Here's how the part is built. I have some questions about the finished solid (model axes, mm). A direction names the side the tool comes from. Coordinates: 2 decimals unless noted, no trailing zeros. Loops run counter-clockwise (first coordinate to the right, second up) from the corner with the lowest first, then second, coordinate; pieces in that order, holes last. Notation, with made-up numbers: M -31,45.5 L 19,45.5 A18 ccw 19,74.5 Z; hole C 37,-16 d2. An arc over 180 degrees is marked long. Use one line per item in the form item = value. Start each with the question number.
(1) Please list where these lines run through material, in increasing order: L1, parallel to X at y = 0.3, z = -0.55; L2, parallel to X at y = -1, z = 1.25; L3, parallel to Y at x = -4.7, z = -0.65.
(2) Imagine slicing it at C-C, the plane y = 0.3. Please give me the cut outline in (x, z), and give its area (3 significant figures).
(3) Thinking about a two-plate mould opening in Y: for faces 1 (the flat face through (0.4, 2.4, 4)), 2 (the flat face through (6.855, -2.158, -1.479)), 3 (the flat face through (0, 2, 7)), which applies, +Y half, -Y half, draft (parallel to the pull), parting line (faces both ways), or undercut?
(4) On a 3-axis mill with a long thin cutter (end or side, diameter ignored), from which of +Z, -Z, +X, -X, +Y, -Y can I reach the whole of each face in a straight line? I mean faces 4 (the flat face through (-6, 1, 0)), 5 (the flat face through (-4, -1.6, -1)), 6 (the flat face through (-1, 2, 1)). Say none if no direction works.
(5) Will these pins go through, and if not, where does the flat tip stop? P1, Ø2.5, axis at x = -4.5, z = -1, coming from the -Y side; P2, Ø1.7, axis at x = 4, y = 0, coming from the +Z side; P3, Ø4, axis at x = 3, z = 4.5, coming from the -Y side.
(6) Imagine slicing it at D-D, the plane z = 3.25. Please give me the cut outline in (x, y).
(7) Imagine slicing it at A-A, the plane x = -4.7. Please give me the cut outline in (y, z), and give its area (3 significant figures).
(8) Imagine slicing it at B-B, the plane z = -1.5. Please give me the cut outline in (x, y).
```python
from build123d import *

# Parameters (mm, degrees)
F1_DEPTH  = 7
F2_W      = 15.6
F2_H      = 6.4
F3_DEPTH  = 3
F5_DEPTH  = 1
F6_SIZE2  = 0.2
F6_SIZE   = 0.6
F8_DEPTH  = 3
F9_R      = 1.1
F10_DEPTH = 3


with BuildPart() as f1:
    # F0 (on Top) → F1 (new body)
    with BuildSketch(Plane.XY):
        with BuildLine():
            Line((-0.4, 2.9), (-0.4, 1.9595917942))
            ThreePointArc((-0.4, 1.9595917942), (0, -2), (0.4, 1.9595917942))
            Line((0.4, 1.9595917942), (0.4, 2.9))
            Line((0.4, 2.9), (5.4, 2.9))
            ThreePointArc((5.4, 2.9), (6.8142135624, 2.3142135624), (7.4, 0.9))
            Line((7.4, 0.9), (7.4, -2.7))
            Line((7.4, -2.7), (7.8, -2.7))
            Line((7.8, -2.7), (7.8, 3.7))
            Line((7.8, 3.7), (-7.8, 3.7))
            Line((-7.8, 3.7), (-7.8, -2.7))
            Line((-7.8, -2.7), (-7.4, -2.7))
            Line((-7.4, -2.7), (-7.4, 0.9))
            ThreePointArc((-7.4, 0.9), (-6.8142135624, 2.3142135624), (-5.4, 2.9))
            Line((-5.4, 2.9), (-0.4, 2.9))
        make_face()
    extrude(amount=F1_DEPTH)

    # F2 (on face) → F3 (join)
    with BuildSketch(Plane(origin=(0, 0, 0), x_dir=(1, 0, 0), z_dir=(0, 0, -1))):
        with Locations((0, -0.5)):
            Rectangle(F2_W, F2_H)
    extrude(amount=F3_DEPTH)

    # F4 (on face) → F5 (join)
    with BuildSketch(Plane.XY):
        with BuildLine():
            Line((-2.7, 2.9), (-2.7, 0))
            ThreePointArc((-2.7, 0), (0, -2.7), (2.7, 0))
            Line((2.7, 0), (2.7, 2.9))
            Line((2.7, 2.9), (-2.7, 2.9))
        make_face()
    extrude(amount=F5_DEPTH)

    # F6
    f6_edges = [f1.edges().sort_by_distance(p)[0] for p in [
        (0, -2.7, 1),
    ]]
    f6_side = f1.faces().sort_by_distance((0, -2.622205, 1))[0]
    chamfer(f6_edges, length=F6_SIZE, length2=F6_SIZE2, reference=f6_side)

    # F7 (on face) → F8 (cut, through all)
    with BuildSketch(Plane.XY):
        with BuildLine():
            ThreePointArc((0, -2.7), (-0.923454387, -2.5371700761), (-1.7355265462, -2.0683199964))
            Line((-1.7355265462, -2.0683199964), (-2.2936485844, -1.6))
            Line((-2.2936485844, -1.6), (-6.7052558883, -1.6))
            Line((-6.7052558883, -1.6), (-7, -2.7))
            Line((-7, -2.7), (0, -2.7))
        make_face()
        with BuildLine():
            ThreePointArc((1.7355265462, -2.0683199964), (0.923454387, -2.5371700761), (0, -2.7))
            Line((0, -2.7), (7, -2.7))
            Line((7, -2.7), (6.7052558883, -1.6))
            Line((6.7052558883, -1.6), (2.2936485844, -1.6))
            Line((2.2936485844, -1.6), (1.7355265462, -2.0683199964))
        make_face()
    extrude(amount=-F8_DEPTH, mode=Mode.SUBTRACT)

    # F9 (on face) → F10 (cut, through all)
    with BuildSketch(Plane(origin=(0, 0, -3), x_dir=(1, 0, 0), z_dir=(0, 0, -1))):
        with Locations((-4.7, -0.3)):
            Circle(F9_R)
        with Locations((4.7, -0.3)):
            Circle(F9_R)
    extrude(amount=-F10_DEPTH, mode=Mode.SUBTRACT)


solid = f1.part
```
Answer:
q1.L1 = -7.8 to -5.8, -3.6 to 3.6, 5.8 to 7.8
q1.L2 = -7.8 to -7.4, -1.73 to 1.73, 7.4 to 7.8
q1.L3 = -1.6 to -0.8, 1.4 to 3.7
q2.outline = M -7.8,-3 L -5.8,-3 L -5.8,0 L -7.4,0 L -7.4,7 L -7.8,7 Z; M -3.6,-3 L 3.6,-3 L 3.6,0 L 2.7,0 L 2.7,0.8 L 2.1,1 L 1.98,1 L 1.98,7 L -1.98,7 L -1.98,1 L -2.1,1 L -2.7,0.8 L -2.7,0 L -3.6,0 Z; M 5.8,-3 L 7.8,-3 L 7.8,7 L 7.4,7 L 7.4,0 L 5.8,0 Z
q2.area = 68.2 mm²
q3.face_1 = undercut
q3.face_2 = -Y half
q3.face_3 = draft
q4.face_4 = +Z, -Y
q4.face_5 = +Z, -Z, -Y
q4.face_6 = +Z
q5.P1 = -1.6
q5.P2 = 0
q5.P3 = -1.73
q6.outline = M -7.8,-2.7 L -7.4,-2.7 L -7.4,0.9 A2 cw -5.4,2.9 L -0.4,2.9 L -0.4,1.96 A2 ccw long 0.4,1.96 L 0.4,2.9 L 5.4,2.9 A2 cw 7.4,0.9 L 7.4,-2.7 L 7.8,-2.7 L 7.8,3.7 L -7.8,3.7 Z
q7.outline = M -1.6,-3 L -0.8,-3 L -0.8,0 L -1.6,0 Z; M 1.4,-3 L 3.7,-3 L 3.7,7 L 2.9,7 L 2.9,0 L 1.4,0 Z
q7.area = 14.9 mm²
q8.outline = M -7.8,-2.7 L -7,-2.7 L -6.71,-1.6 L -2.29,-1.6 L -1.74,-2.07 A2.7 ccw 1.74,-2.07 L 2.29,-1.6 L 6.71,-1.6 L 7,-2.7 L 7.8,-2.7 L 7.8,3.7 L -7.8,3.7 Z; hole C -4.7,0.3 d2.2; hole C 4.7,0.3 d2.2
